Can you work these out from the drawing? Everything is in mm from the part's minimum corner. Round coordinates to 2 decimals unless told otherwise and drop trailing zeros. Write each loop counter-clockwise with the first axis right and the second up, starting at its lowest first coordinate (ties: lowest second). Pieces come first, ordered by that corner, then holes. Notation, with made-up numbers: (28, 72.25) -> (61, 72.25) arc R16 ccw to (61, 82.25) -> close; hole circle Ø11 at (75, -38.75). An arc over 180 degrees is marked (long way). Answer as CSV lines item,"result". Start each with the question number.
Q1. If I drill on line 1 (X direction, y = 12, z = 6); line 2 (Z direction, x = 31.3, y = 20); line 3 (Z direction, x = 23.5, y = 18), over which ranges is the centre line in solid material (lowest first)? Write a range as [from, to].
Q2. Imagine slicing it at D-D on y = 25.5. Please give me the cut outline in (x, z).
Q3. Imagine slicing it at B-B on x = 20. Please give me the cut outline in (y, z), and give its area (3 significant figures).
Q4. Imagine slicing it at C-C on z = 38. Please give me the cut outline in (x, y), and give its area (3 significant figures).
Q5. Imagine slicing it at A-A on z = 12. Please give me the cut outline in (x, y), and give its area (3 significant figures).
Q6. If we mould it in two halves opening along X, with no side actions, what happens to the marked faces 1, 2 and 3? For each: pulls with the +X half, pulls with the -X half, needs draft (parallel to the pull), parting line crosses it, or undercut.
Q7. Will these pins go through, and if not, where does the flat tip stop? pin 1 Ø5 at (x, y) = (21, 25.5) entering from +Z; pin 2 Ø1.5 at (x, y) = (26.5, 34) entering from -Z; pin 3 Ø6 at (y, z) = (18.5, 19.5) entering from -X; pin 4 Ø4 at (x, y) = (20.5, 22.5) entering from -Z.
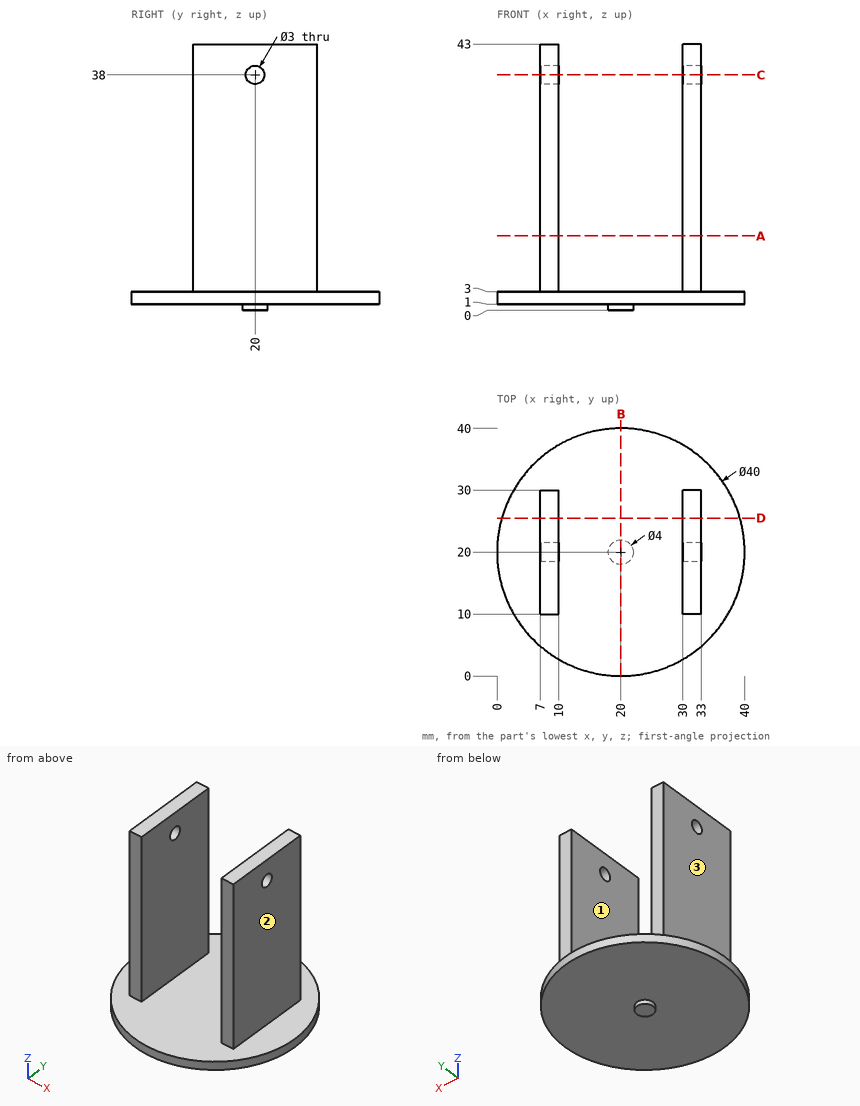
Checks:
1,line 1,"[7, 10], [30, 33]"
1,line 2,"[1, 36.5], [39.5, 43]"
1,line 3,"[1, 3]"
2,outline,"(0.77, 1) -> (39.23, 1) -> (39.23, 3) -> (33, 3) -> (33, 43) -> (30, 43) -> (30, 3) -> (10, 3) -> (10, 43) -> (7, 43) -> (7, 3) -> (0.77, 3) -> close"
3,outline,"(0, 1) -> (18, 1) -> (18, 0) -> (22, 0) -> (22, 1) -> (40, 1) -> (40, 3) -> (0, 3) -> close"
3,area,"84.0 mm^2"
4,outline,"(7, 10) -> (10, 10) -> (10, 18.5) -> (7, 18.5) -> close; (7, 21.5) -> (10, 21.5) -> (10, 30) -> (7, 30) -> close; (30, 10) -> (33, 10) -> (33, 18.5) -> (30, 18.5) -> close; (30, 21.5) -> (33, 21.5) -> (33, 30) -> (30, 30) -> close"
4,area,"102 mm^2"
5,outline,"(7, 10) -> (10, 10) -> (10, 30) -> (7, 30) -> close; (30, 10) -> (33, 10) -> (33, 30) -> (30, 30) -> close"
5,area,"120 mm^2"
6,face 1,"undercut"
6,face 2,"pulls with the +X half"
6,face 3,"pulls with the -X half"
7,pin 1,"z = 3"
7,pin 2,"z = 1"
7,pin 3,"x = 7"
7,pin 4,"z = 0"
